```python
from build123d import *

# Parameters (mm, degrees)
ESTRUSIONE_ESTRUSIONE1_DEPTH = 2
TAGLIO_ESTRUSIONE1_DEPTH     = 69.058798109
SCHIZZO3_R                   = 1.5
TAGLIO_ESTRUSIONE3_DEPTH     = 69.058798109
ESTRUSIONE_ESTRUSIONE2_DEPTH = 2


with BuildPart() as part:
    # Schizzo1 → Estrusione-Estrusione1 (new body)
    with BuildSketch(Plane.XY):
        Polygon((0, 0), (0, -62), (10, -62), (10, -14), (28, -14), (28, 0), align=None)
    extrude(amount=-ESTRUSIONE_ESTRUSIONE1_DEPTH)

    # Schizzo2 → Taglio-Estrusione1 (cut, through all)
    with BuildSketch(Plane.XY):
        Polygon((3, -62), (0, -58), (0, -62), align=None)
        Polygon((10, -58), (7, -62), (10, -62), align=None)
        Polygon((0, -4), (3, 0), (0, 0), align=None)
        Polygon((25, 0), (28, 0), (28, -4), align=None)
        Polygon((28, -14), (25, -14), (28, -10), align=None)
    extrude(amount=-TAGLIO_ESTRUSIONE1_DEPTH, mode=Mode.SUBTRACT)

    # Schizzo3 → Taglio-Estrusione3 (cut, through all)
    with BuildSketch(Plane.XY):
        with Locations((5, -8)):
            Circle(SCHIZZO3_R)
        with Locations((22, -8)):
            Circle(SCHIZZO3_R)
        with Locations((5, -58)):
            Circle(SCHIZZO3_R)
    extrude(amount=-TAGLIO_ESTRUSIONE3_DEPTH, mode=Mode.SUBTRACT)

    # Schizzo4 → Estrusione-Estrusione2 (add)
    with BuildSketch(Plane.XY):
        with BuildLine():
            Line((10, -21.5), (10, -14))
            Line((10, -14), (17.5, -14))
            ThreePointArc((17.5, -14), (12.196699141, -16.196699141), (10, -21.5))
        make_face()
    extrude(amount=-ESTRUSIONE_ESTRUSIONE2_DEPTH)


solid = part.part
```
Here's how the part is built. I have some questions about the finished solid (model axes, mm). A direction names the side the tool comes from. Coordinates: 2 decimals unless noted, no trailing zeros. Order: outer loops, then holes, each group sorted by start corner. A loop starts at its lowest first (then second) coordinate and runs counter-clockwise, first axis right, second up. Notation, with made-up numbers: (-20.5, -7) - (-12.5, -7) arc R14 ccw to (-12.5, 4) - close; hole circle Ø1 at (78.5, 72.5). An arc over 180 degrees is marked (long way). One line per question, with ' | ' between items.
(1) For faces 1 (the flat face through (10, -40, -1)), 2 (the flat face through (5, -62, -1)), which set-ups out of +Z, -Z, +X, -X, +Y, -Y let a thin tool reach every point of the face, with its end or its side?
Report:
face 1: +Z, -Z, +X, -Y | face 2: +Z, -Z, +X, -X, -Y
(2) If I drill on L1, parallel to Y at x = 5, z = -0.95; L2, parallel to Y at x = 22, z = -1.2; L3, parallel to Y at x = 4.25, z = -1.75, over which ranges is the centre line in solid material (lowest first)?
Report:
L1: y = -62 to -59.5, -56.5 to -9.5, -6.5 to 0 | L2: y = -14 to -9.5, -6.5 to 0 | L3: y = -62 to -59.3, -56.7 to -9.3, -6.7 to 0
(3) Suppose I cut it at D-D on x = 5. List the corners of the cut face in (y, z) for me, and give its area (3 significant figures).
Report:
outline: (-62, -2) - (-59.5, -2) - (-59.5, 0) - (-62, 0) - close; (-56.5, -2) - (-9.5, -2) - (-9.5, 0) - (-56.5, 0) - close; (-6.5, -2) - (0, -2) - (0, 0) - (-6.5, 0) - close | area: 112 mm2
(4) Suppose I cut it at B-B on y = -8. List the corners of the cut face in (x, z) for me.
Report:
outline: (0, -2) - (3.5, -2) - (3.5, 0) - (0, 0) - close; (6.5, -2) - (20.5, -2) - (20.5, 0) - (6.5, 0) - close; (23.5, -2) - (28, -2) - (28, 0) - (23.5, 0) - close
(5) Suppose I cut it at C-C on z = -0.4. List the corners of the cut face in (x, y) for me, and give its area (3 significant figures).
Report:
outline: (0, -58) - (3, -62) - (7, -62) - (10, -58) - (10, -21.5) arc R7.5 cw to (17.5, -14) - (25, -14) - (28, -10) - (28, -4) - (25, 0) - (3, 0) - (0, -4) - close; hole circle Ø3 at (5, -58); hole circle Ø3 at (5, -8); hole circle Ø3 at (22, -8) | area: 833 mm2
(6) If we mould it in two halves opening along Y, with no side actions, what happens to faces 3 (the flat face through (14, 0, -1)), 4 (the flat face through (28, -7, -1)), 5 (the cylindrical face through (4.805, -56.513, -0.986))? For each: pulls with the +Y half, pulls with the -Y half, needs draft (parallel to the pull), parting line crosses it, or undercut.
Report:
face 3: pulls with the +Y half | face 4: needs draft | face 5: undercut
(7) Suppose I cut it at A-A on x = 22. List the corners of the cut face in (y, z) for me, and give its area (3 significant figures).
Report:
outline: (-14, -2) - (-9.5, -2) - (-9.5, 0) - (-14, 0) - close; (-6.5, -2) - (0, -2) - (0, 0) - (-6.5, 0) - close | area: 22.0 mm2
(8) Will this pin go through, and if not, where does the flat tip stop? pin 1 (2.5 mm diameter, centred on x = 5, y = -8, fed in from +Z).
Report:
pin 1: passes through
